from build123d import *

# Parameters (mm, degrees)
F0_W     = 9
F0_H     = 9
F0_R     = 3.5
F0_R_2   = 2.1
F1_DEPTH = 8
F2_R     = 4
F2_R_2   = 2.1
F3_DEPTH = 6
F4_R     = 1
F5_R     = 6.9957101535
F5_R_2   = 4.3441334804
F6_DEPTH = 25


with BuildPart() as f1:
    # F0 (on Top) → F1 (new body)
    with BuildSketch(Plane.XY):
        Rectangle(F0_W, F0_H)
        Circle(F0_R, mode=Mode.SUBTRACT)
        Circle(F0_R)
        Circle(F0_R_2, mode=Mode.SUBTRACT)
    extrude(amount=F1_DEPTH)

    # F2 (on face) → F3 (cut)
    with BuildSketch(Plane(origin=(0, 0, 0), x_dir=(1, 0, 0), z_dir=(0, 0, -1))):
        Circle(F2_R)
        Circle(F2_R_2, mode=Mode.SUBTRACT)
    extrude(amount=-F3_DEPTH, mode=Mode.SUBTRACT)

    # F4
    f4_edges = [f1.edges().sort_by_distance(p)[0] for p in [
        (-4, 0, 6),
    ]]
    fillet(f4_edges, radius=F4_R)

    # F5 (on face) → F6 (cut)
    with BuildSketch(Plane(origin=(0, 0, 0), x_dir=(1, 0, 0), z_dir=(0, 0, -1))):
        Circle(F5_R)
        Circle(F5_R_2, mode=Mode.SUBTRACT)
    extrude(amount=-F6_DEPTH, mode=Mode.SUBTRACT)


solid = f1.part
Verification items for the finished model (mm, model axes). Give positions to 0.01 mm unless a question says otherwise; leave off trailing zeros. Loops run counter-clockwise (first coordinate to the right, second up) from the corner with the lowest first, then second, coordinate; pieces in that order, holes last.
1) Thickness scan on line 1 along Y through (x, z) = (0, 2.2); line 2 along X through (y, z) = (0, 7); line 3 along Z through (x, y) = (1.75, -1.5). Record the ranges inside material, lowest first.
2) Sectioned sample at C-C, the plane z = 2. Enter the section's corners in (x, y).
3) Draft check along Y on faces 1 (the cylindrical face through (-3.2, -2.94, 3.94)), 2 (the cylindrical face through (-0.867, 3.905, 2.465)), 3 (the flat face through (1.3, 2, 6)). Enter one of: pulls with the +Y half, pulls with the -Y half, needs draft (parallel to the pull), parting line crosses it, or undercut.
4) Sectioned sample at D-D, the plane z = 7.25. Enter the section's corners in (x, y), then the cut area to 3 significant figures.
5) Depth check by flat-ended pin: pin 1 Ø2 at (x, z) = (-2.5, 1) entering from -Y; pin 2 Ø1 at (x, z) = (3, 1.5) entering from +Y; pin 3 Ø1.5 at (x, y) = (1, -0.5) entering from +Z; pin 4 Ø5 at (x, y) = (-1, -0.5) entering from -Z. Enter the tip coordinate at first touch or a pass-through.
6) Sectioned sample at A-A, the plane y = 0. Enter the section's corners in (x, z).
Answers:
1. line 1: y = -4.34 to -4, 4 to 4.34
1. line 2: x = -4.34 to -2.1, 2.1 to 4.34
1. line 3: z = 6 to 8
2. outline: circle Ø8.69 at (0, 0); hole circle Ø8 at (0, 0)
3. face 1: parting line crosses it
3. face 2: undercut
3. face 3: undercut
4. outline: circle Ø8.69 at (0, 0); hole circle Ø4.2 at (0, 0)
4. area: 45.4 mm2
5. pin 1: stops at y = -4.08
5. pin 2: stops at y = 3.55
5. pin 3: passes through
5. pin 4: stops at z = 5.79
6. outline: (-4.34, 0) - (-4, 0) - (-4, 5) arc R1 cw to (-3, 6) - (-2.1, 6) - (-2.1, 8) - (-4.34, 8) - close; (2.1, 6) - (3, 6) arc R1 cw to (4, 5) - (4, 0) - (4.34, 0) - (4.34, 8) - (2.1, 8) - close
